Verification items for the finished model (mm, model axes). A direction names the side the tool comes from. Round coordinates to 2 decimals unless told otherwise and drop trailing zeros.
from build123d import *

# Parameters (mm, degrees)
F1_R     = 20
F1_R_2   = 0.675
F2_DEPTH = 4.5
F3_R     = 20
F3_R_2   = 18
F4_DEPTH = 2
F5_R     = 16.25
F5_R_2   = 13.75
F5_R_3   = 5
F5_R_4   = 2.5
F6_DEPTH = 0.3
F7_R     = 0.5


with BuildPart() as f2:
    # F1 (on face) → F2 (new body)
    with BuildSketch(Plane.XY):
        Circle(F1_R)
        with Locations((-9.5262794416, -5.5)):
            Circle(F1_R_2, mode=Mode.SUBTRACT)
        with Locations((-3.5, -6.0621778265)):
            Circle(F1_R_2, mode=Mode.SUBTRACT)
        with Locations((0, -11)):
            Circle(F1_R_2, mode=Mode.SUBTRACT)
        with Locations((3.5, -6.0621778265)):
            Circle(F1_R_2, mode=Mode.SUBTRACT)
        with Locations((9.5262794416, -5.5)):
            Circle(F1_R_2, mode=Mode.SUBTRACT)
        with Locations((-7, 0)):
            Circle(F1_R_2, mode=Mode.SUBTRACT)
        with Locations((-9.5262794416, 5.5)):
            Circle(F1_R_2, mode=Mode.SUBTRACT)
        with Locations((-3.5, 6.0621778265)):
            Circle(F1_R_2, mode=Mode.SUBTRACT)
        Circle(F1_R_2, mode=Mode.SUBTRACT)
        with Locations((7, 0)):
            Circle(F1_R_2, mode=Mode.SUBTRACT)
        with Locations((3.5, 6.0621778265)):
            Circle(F1_R_2, mode=Mode.SUBTRACT)
        with Locations((9.5262794416, 5.5)):
            Circle(F1_R_2, mode=Mode.SUBTRACT)
        with Locations((0, 11)):
            Circle(F1_R_2, mode=Mode.SUBTRACT)
    extrude(amount=F2_DEPTH)

    # F3 (on face) → F4 (join)
    with BuildSketch(Plane.XY.offset(4.5)):
        Circle(F3_R)
        Circle(F3_R_2, mode=Mode.SUBTRACT)
    extrude(amount=F4_DEPTH)

    # F5 (on face) → F6 (cut)
    with BuildSketch(Plane.XY):
        Circle(F5_R)
        Circle(F5_R_2, mode=Mode.SUBTRACT)
        Circle(F5_R_3)
        Circle(F5_R_4, mode=Mode.SUBTRACT)
    extrude(amount=F6_DEPTH, mode=Mode.SUBTRACT)

    # F7
    f7_edges = [f2.edges().sort_by_distance(p)[0] for p in [
        (-20, 0, 0),
    ]]
    fillet(f7_edges, radius=F7_R)


solid = f2.part
Q1. Release check for a two-part mould opening along Y. For faces 1 (the flat face through (6, 0, 0)), 2 (the cylindrical face through (0.31, 10.4, 2.22)) record: released by +Y, released by -Y, zero draft, split by the parting line, or undercut.
Recorded:
face 1: zero draft
face 2: undercut
Q2. Sectioned sample at A-A (y = 0). Give the number of separate pieces and of enclosed holes in the cut face, plus the area to 3 significant figures.
Recorded:
separate pieces: 4
enclosed holes: 0
area: 167 mm2
Q3. Tool access check on faces 3 (the flat face through (2, -2, 0.3)), 4 (the cylindrical face through (0.31, -11.6, 2.22)). Record the directions out of +Z, -Z, +X, -X, +Y, -Y that give a thin tool (end or side, any length) a straight path to the whole face; none if there is none.
Recorded:
face 3: -Z
face 4: +Z, -Z
Q4. Material ranges on line 1 along Y through (x, z) = (0, 2) (3 decimals); line 2 along Y through (x, z) = (-3.5, 3.45); line 3 along Y through (x, z) = (4, 3), recorded low to high.
Recorded:
line 1: y = -20 to -11.675, -10.325 to -0.675, 0.675 to 10.325, 11.675 to 20
line 2: y = -19.69 to -6.74, -5.39 to 5.39, 6.74 to 19.69
line 3: y = -19.6 to -6.52, -5.61 to 5.61, 6.52 to 19.6
Q5. Depth check by flat-ended pin: P1, Ø1.6, axis at x = -9.53, y = -5.5, coming from the +Z side; P2, Ø1, axis at x = -5, z = 3.5, coming from the -Y side; P3, Ø1, axis at x = 6.5, z = 4.5, coming from the -Y side; P4, Ø1.2, axis at x = -7, y = 0, coming from the -Z side. Enter the tip coordinate at first touch or a pass-through.
Recorded:
P1: stops at z = 4.5
P2: stops at y = -19.49
P3: stops at y = -19.08
P4: passes through
